from build123d import *

# Parameters (mm, degrees)
F1_DEPTH  = 7.5
F2_T      = -1.5
F4_DEPTH  = 7.5
F6_DEPTH  = 3
F7_R      = 3.25
F8_DEPTH  = 32.25
F9_R      = 3.25
F10_DEPTH = 50.001


with BuildPart() as f1:
    # F0 (on Top) → F1 (new body)
    with BuildSketch(Plane.XY):
        Polygon((25, -8.75), (25, 8.75), (8.75, 8.75), (-8.75, 8.75), (-25, 8.75), (-25, -8.75), (-8.75, -8.75), (-8.75, -25), (0, -25), (8.75, -25), (8.75, -8.75), align=None)
    extrude(amount=F1_DEPTH)

    # F2
    f2_openings = [f1.faces().sort_by_distance(p)[0] for p in [
        (0, -4.139151, 7.5),
    ]]
    offset(amount=F2_T, openings=f2_openings, kind=Kind.INTERSECTION)

    # F3 (on face) → F4 (join, through all)
    with BuildSketch(Plane.XY.offset(7.5)):
        Polygon((-23.5, 7.25), (-23.5, 4.4215728753), (-20.6715728753, 7.25), align=None)
        Polygon((-8.75, -8.75), (-11.5784271247, -8.75), (-8.75, -11.5784271247), align=None)
        Polygon((23.5, 7.25), (20.6715728753, 7.25), (23.5, 4.4215728753), align=None)
        Polygon((8.75, -11.5784271247), (11.5784271247, -8.75), (8.75, -8.75), align=None)
    extrude(amount=-F4_DEPTH)

    # F5 (on face) → F6 (cut)
    with BuildSketch(Plane.XY.offset(7.5)):
        with BuildLine():
            ThreePointArc((-9.6338834765, -9.6338834765), (-8.8165408163, -9.79646304), (-8.3535533906, -9.1035533906))
            ThreePointArc((-8.3535533906, -9.1035533906), (-9.3905659649, -8.4106437412), (-9.6338834765, -9.6338834765))
        make_face()
        with BuildLine():
            ThreePointArc((-22.6161165235, 6.3661165235), (-22.45353696, 6.6094340351), (-22.3964466094, 6.8964466094))
            ThreePointArc((-22.3964466094, 6.8964466094), (-23.8393562588, 7.1834591837), (-22.6161165235, 6.3661165235))
        make_face()
        with BuildLine():
            ThreePointArc((9.6338834765, -9.6338834765), (9.79646304, -9.3905659649), (9.8535533906, -9.1035533906))
            ThreePointArc((9.8535533906, -9.1035533906), (8.4106437412, -8.8165408163), (9.6338834765, -9.6338834765))
        make_face()
        with BuildLine():
            ThreePointArc((22.6161165235, 6.3661165235), (23.4334591837, 6.20353696), (23.8964466094, 6.8964466094))
            ThreePointArc((23.8964466094, 6.8964466094), (22.8594340351, 7.5893562588), (22.6161165235, 6.3661165235))
        make_face()
    extrude(amount=-F6_DEPTH, mode=Mode.SUBTRACT)

    # F7 (on face) → F8 (cut, through all)
    with BuildSketch(Plane.XZ.offset(25)):
        with Locations((0, 7.5)):
            Circle(F7_R)
    extrude(amount=-F8_DEPTH, mode=Mode.SUBTRACT)

    # F9 (on face) → F10 (cut, through all)
    with BuildSketch(Plane(origin=(-25, 0, 0), x_dir=(0, -1, 0), z_dir=(-1, 0, 0))):
        with Locations((0, 7.5)):
            Circle(F9_R)
    extrude(amount=-F10_DEPTH, mode=Mode.SUBTRACT)


solid = f1.part
Read the model definition and answer for the solid it produces. Units are mm, in the model's axes. A direction names the side the tool comes from. Give positions to 0.01 mm unless a question says otherwise; leave off trailing zeros. Loops run counter-clockwise (first coordinate to the right, second up) from the corner with the lowest first, then second, coordinate; pieces in that order, holes last. Notation, with made-up numbers: (79, -13) -> (96, -13) arc R16 ccw to (96, -5) -> close; hole circle Ø7 at (-2, -21.5). An arc over 180 degrees is marked (long way). Answer as CSV lines item,"result".
Item 1: Find section A-A on x = 0. Give the vertices of the cut face in (y, z), plus the area to 4 significant figures.
Returned:
outline,"(-25, 0) -> (8.75, 0) -> (8.75, 7.5) -> (7.25, 7.5) -> (7.25, 1.5) -> (-23.5, 1.5) -> (-23.5, 4.25) -> (-25, 4.25) -> close"
area,"63.75 mm²"
Item 2: Consider line 1 (Y direction, x = -6.5, z = 6); line 2 (Y direction, x = -8, z = 6.75); line 3 (X direction, y = -23, z = 5.75). Determine where each line is inside the solid, lowest interval first. Write a range as [from, to].
Returned:
line 1,"y = [-25, -23.5], [7.25, 8.75]"
line 2,"y = [-25, -7.25], [7.25, 8.75]"
line 3,"x = [-8.75, -7.25], [7.25, 8.75]"
Item 3: Find section B-B on y = -6. Give the vertices of the cut face in (x, z).
Returned:
outline,"(-25, 0) -> (25, 0) -> (25, 7.5) -> (23.5, 7.5) -> (23.5, 1.5) -> (-23.5, 1.5) -> (-23.5, 7.5) -> (-25, 7.5) -> close"
Item 4: Determine the mould class of faces 1 (the face through (-7.25, -15, 4)), 2 (the face through (0, -25, 4)), 3 (the face through (-10.184, -10.144, 3.802)), 4 (the face through (-22.106, 5.816, 4.542)) for opening direction X: +X half, -X half, draft (parallel to the pull), parting line (faces both ways), or undercut.
Returned:
face 1,"undercut"
face 2,"draft"
face 3,"-X half"
face 4,"undercut"
Item 5: Each of these flat-tipped pins is pushed along its axis until it touches: pin 1 (1 mm diameter, centred on x = -17.5, z = 6, fed in from -Y); pin 2 (4 mm diameter, centred on x = 7.5, y = -2, fed in from +Z); pin 3 (2 mm diameter, centred on x = -9.1, y = -9.1, fed in from +Z); pin 4 (1.5 mm diameter, centred on y = -19, z = 3.5, fed in from +X). Where does it stop, or does it pass through?
Returned:
pin 1,"stops at y = -8.75"
pin 2,"stops at z = 1.5"
pin 3,"stops at z = 7.5"
pin 4,"stops at x = 8.75"
Item 6: Find section D-D on z = 6. State how many separate pieces and enclosed holes the cut face has, plus the area to 3 significant figures.
Returned:
separate pieces,"3"
enclosed holes,"4"
area,"225 mm²"
Item 7: For faces 5 (the face through (-18, -8.75, 4)), 6 (the face through (8.75, -18, 4)), 7 (the face through (-9, -9, 4.5)), determine the directions among +Z, -Z, +X, -X, +Y, -Y from which every point of the face is accessible in a straight line to the end or side of a thin tool.
Returned:
face 5,"+Z, -Z, -X, -Y"
face 6,"+Z, -Z, +X, -Y"
face 7,"+Z"
Item 8: Find section C-C on z = 1. Give the vertices of the cut face in (x, y), plus the area to 3 significant figures.
Returned:
outline,"(-25, -8.75) -> (-11.58, -8.75) -> (-8.75, -11.58) -> (-8.75, -25) -> (8.75, -25) -> (8.75, -11.58) -> (11.58, -8.75) -> (25, -8.75) -> (25, 8.75) -> (-25, 8.75) -> close"
area,"1,170 mm²"
